```python
from build123d import *

# Parameters (mm, degrees)
F1_DEPTH    = 100
F2_T1_DEPTH = 125
F2_T3_DEPTH = 124.4948974279
F3_T1_DEPTH = 124.4948974279
F3_T3_DEPTH = 125
F5_D        = 8
F7_R        = 7.5
F10_DEPTH   = 25
F14_DEPTH   = 25


# Not quite as in the source:
# - a fillet or chamfer that OpenCascade refuses, or shapes differently, is made with other operations: its cross-section is extruded or revolved along the edge and cut away or added


with BuildPart() as f1:
    # F0 (on Front) → F1 (new body)
    with BuildSketch(Plane.XZ):
        Polygon((140, 0), (0, 0), (0, -15), (4, -15), (4, -4), (136, -4), (136, -15), (140, -15), align=None)
    extrude(amount=F1_DEPTH)

    # F2: fillet of radius 5 on 2 edges, made by hand

    # F2_s2 → F2_t1 (cut)
    with BuildSketch(Plane.XZ.offset(-12.5)):
        with BuildLine():
            ThreePointArc((5, 0), (1.4644660941, -1.4644660941), (0, -5))
            Line((0, -5), (0, 0))
            Line((0, 0), (5, 0))
        make_face()
    extrude(amount=F2_T1_DEPTH, mode=Mode.SUBTRACT)

    # F2_s4 → F2_t3 (cut)
    with BuildSketch(Plane.XZ.offset(-12.2474487139)):
        with BuildLine():
            ThreePointArc((136, -15), (138.8729833462, -13.2632981746), (140, -10.1010205144))
            Line((140, -10.1010205144), (140, -15))
            Line((140, -15), (136, -15))
        make_face()
    extrude(amount=F2_T3_DEPTH, mode=Mode.SUBTRACT)

    # F3: fillet of radius 5 on 2 edges, made by hand

    # F3_s2 → F3_t1 (cut)
    with BuildSketch(Plane.XZ.offset(-12.2474487139)):
        with BuildLine():
            ThreePointArc((4, -15), (1.1270166538, -13.2632981746), (0, -10.1010205144))
            Line((0, -10.1010205144), (0, -15))
            Line((0, -15), (4, -15))
        make_face()
    extrude(amount=F3_T1_DEPTH, mode=Mode.SUBTRACT)

    # F3_s4 → F3_t3 (cut)
    with BuildSketch(Plane.XZ.offset(-12.5)):
        with BuildLine():
            ThreePointArc((135, 0), (138.5355339059, -1.4644660941), (140, -5))
            Line((140, -5), (140, 0))
            Line((140, 0), (135, 0))
        make_face()
    extrude(amount=F3_T3_DEPTH, mode=Mode.SUBTRACT)

    # F5 (through all)
    with Locations(Plane.XY):
        with Locations((25, -20), (115, -20), (25, -80), (115, -80)):
            Hole(F5_D / 2)

    # F9 (on Right) → F10 (join, symmetric)
    with BuildSketch(Plane.YZ):
        with BuildLine():
            Line((0, 5), (0, 0))
            Line((0, 0), (0, -5))
            Line((0, -5), (0, -15))
            ThreePointArc((0, -15), (10, -5), (0, 5))
        make_face()
    extrude(amount=F10_DEPTH, both=True)

    # F13 (on offset) → F14 (join, symmetric)
    with BuildSketch(Plane.YZ.offset(140)):
        with BuildLine():
            Line((0, -10.1010205144), (0, -15))
            ThreePointArc((0, -15), (10, -5), (0, 5))
            Line((0, 5), (0, 0))
            Line((0, 0), (0, -5))
            Line((0, -5), (0, -10.1010205144))
        make_face()
    extrude(amount=F14_DEPTH, both=True)


with BuildPart() as f8:
    # F8: sweep along a path in F6
    with BuildLine(Plane.XZ) as f8_path:
        Line((-40, 0), (-40, 100))
        ThreePointArc((-40, 100), (-85, 150), (-130, 100))
        Line((-130, 100), (-130, 0))
    # F7 (on Top) → F8 (sweep)
    with BuildSketch(Plane.XY):
        with Locations((-40, 0)):
            Circle(F7_R)
    sweep(path=f8_path.line)


solid = f1.part
```
Could you check a few things on this model? Use its own coordinates, in mm. A direction names the side the tool comes from. Coordinates: 2 decimals unless noted, no trailing zeros. Write each loop counter-clockwise with the first axis right and the second up, starting at its lowest first coordinate (ties: lowest second). Pieces come first, ordered by that corner, then holes. Notation, with made-up numbers: (41, 45) -> (72, 45) arc R11 cw to (72, 61) -> close; hole circle Ø6 at (53, 58). An arc over 180 degrees is marked (long way). Return JSON: item names as keys, results as strings.
(1) We'd pull the mould along Y, two halves only. Please class faces 1 (the cylindrical face through (140, 10, -5)), 2 (the cylindrical face through (113.154, -83.549, -2.028)), 3 (the flat face through (69, -49, -4)): +Y half, -Y half, draft (parallel to the pull), parting line (faces both ways), or undercut.
Numbers:
{"face 1": "+Y half", "face 2": "undercut", "face 3": "draft"}
(2) Imagine slicing it at D-D, the plane x = 61. Please give me the cut outline in (y, z).
Numbers:
{"outline": "(-100, -4) -> (0, -4) -> (0, 0) -> (-100, 0) -> close"}
(3) I'm going to push flat-ended pins straight in: pin 1 (1.5 mm diameter, centred on y = -61.5, z = -7.5, fed in from -X); pin 2 (2 mm diameter, centred on x = 75.5, z = -2.5, fed in from +Y); pin 3 (6 mm diameter, centred on x = 66.5, y = -64.5, fed in from +Z). Where does each tip first touch, or does it pass through?
Numbers:
{"pin 1": "stops at x = 0", "pin 2": "stops at y = 0", "pin 3": "stops at z = 0"}
(4) Imagine slicing it at A-A, the plane y = -80. Please give me the cut outline in (x, z), then the cut area to 3 significant figures.
Numbers:
{"outline": "(0, -10.1) arc R5 ccw to (4, -15) -> (4, -4) -> (21, -4) -> (21, 0) -> (5, 0) arc R5 ccw to (0, -5) -> close; (29, -4) -> (111, -4) -> (111, 0) -> (29, 0) -> close; (119, -4) -> (136, -4) -> (136, -15) arc R5 ccw to (140, -10.1) -> (140, -5) arc R5 ccw to (135, 0) -> (119, 0) -> close", "area": "563 mm2"}
(5) Imagine slicing it at B-B, the plane z = -12.25. Please give me the cut outline in (x, y).
Numbers:
{"outline": "(-25, 0) -> (0.49, 0) -> (0.49, -100) -> (4, -100) -> (4, 0) -> (25, 0) -> (25, 6.89) -> (-25, 6.89) -> close; (115, 0) -> (136, 0) -> (136, -100) -> (139.51, -100) -> (139.51, 0) -> (165, 0) -> (165, 6.89) -> (115, 6.89) -> close"}
(6) Imagine slicing it at C-C, the plane y = -50. Please give me the cut outline in (x, z).
Numbers:
{"outline": "(0, -10.1) arc R5 ccw to (4, -15) -> (4, -4) -> (136, -4) -> (136, -15) arc R5 ccw to (140, -10.1) -> (140, -5) arc R5 ccw to (135, 0) -> (5, 0) arc R5 ccw to (0, -5) -> close"}
(7) Which directions (+Z, -Z, +X, -X, +Y, -Y) give clear straight access to the entire face, cutting with the end or side of a thin tool? Please do faces 4 (the cylindrical face through (2, -49, -1)), 5 (the cylindrical face through (138, -49, -1)), 6 (the flat face through (25, 4, -5)), 7 (the flat face through (71, -49, 0)).
Numbers:
{"face 4": "+Z, -X, -Y", "face 5": "+Z, +X, -Y", "face 6": "+Z, -Z, +Y", "face 7": "+Z, +X, -X, -Y"}
(8) I need wall thicknesses on L1, parallel to X at y = -67, z = -7.25; L2, parallel to Z at x = 62, y = -12.5; L3, parallel to X at y = -25, z = -13.25. Which ranges of each line are inside material? Lowest first, please.
Numbers:
{"L1": "x = 0 to 4, 136 to 140", "L2": "z = -4 to 0", "L3": "x = 1.12 to 4, 136 to 138.88"}
